from build123d import *

# Parameters (mm, degrees)
SKETCH1_W           = 32
SKETCH1_H           = 32
BOSS_EXTRUDE1_DEPTH = 5
BOSS_EXTRUDE2_DEPTH = 30
SKETCH3_R           = 5
SKETCH3_R_2         = 2
CUT_EXTRUDE1_DEPTH  = 10
SKETCH4_R           = 2
CUT_EXTRUDE2_DEPTH  = 58.210138962


with BuildPart() as part:
    # Sketch1 → Boss-Extrude1 (new body)
    with BuildSketch(Plane(origin=(0, 0, 0), x_dir=(1, 0, 0), z_dir=(0, 1, 0))):
        with Locations((0, -16)):
            Rectangle(SKETCH1_W, SKETCH1_H)
    extrude(amount=BOSS_EXTRUDE1_DEPTH)

    # Sketch2 → Boss-Extrude2 (add)
    with BuildSketch(Plane(origin=(0, 5, 0), x_dir=(1, 0, 0), z_dir=(0, 1, 0))):
        with BuildLine():
            Line((-16, -7), (-11.720842953, -7))
            ThreePointArc((-11.720842953, -7), (-11.587559316, -8.18927833), (-11, -9.231833616))
            Line((-11, -9.231833616), (-11, -22.772628888))
            ThreePointArc((-11, -22.772628888), (-11.586870055, -23.813052847), (-11.721238688, -25))
            Line((-11.721238688, -25), (-16, -25))
            Line((-16, -25), (-16, -7))
        make_face()
        with BuildLine():
            Line((16, -25), (11.725701193, -25))
            ThreePointArc((11.725701193, -25), (11.590282481, -23.809816196), (11, -22.767490763))
            Line((11, -22.767490763), (11, -9.236971742))
            ThreePointArc((11, -9.236971742), (11.590974158, -8.192515764), (11.725305458, -7))
            Line((11.725305458, -7), (16, -7))
            Line((16, -7), (16, -25))
        make_face()
    extrude(amount=BOSS_EXTRUDE2_DEPTH)

    # Sketch3 → Cut-Extrude1 (cut)
    with BuildSketch(Plane.XZ):
        with Locations(Location((0, 16, 0), (0, 0, 270))):
            Circle(SKETCH3_R)
        with Locations(Location((-8.732768748, 7.267231252, 0), (0, 0, 270))):
            Circle(SKETCH3_R_2)
        with Locations(Location((-8.732768748, 24.732768748, 0), (0, 0, 270))):
            Circle(SKETCH3_R_2)
        with Locations(Location((8.732768748, 24.732768748, 0), (0, 0, 270))):
            Circle(SKETCH3_R_2)
        with Locations(Location((8.732768748, 7.267231252, 0), (0, 0, 270))):
            Circle(SKETCH3_R_2)
    extrude(amount=-CUT_EXTRUDE1_DEPTH, mode=Mode.SUBTRACT)

    # Sketch4 → Cut-Extrude2 (cut, through all)
    with BuildSketch(Plane.ZY.offset(16)):
        with Locations((16, 23.5)):
            Circle(SKETCH4_R)
    extrude(amount=-CUT_EXTRUDE2_DEPTH, mode=Mode.SUBTRACT)


solid = part.part
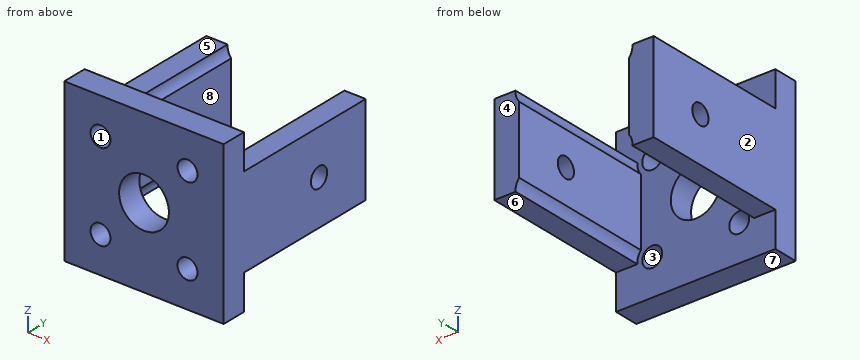
The listing builds one solid part. Answer for the finished solid, in the listing's coordinates (mm). Face numbers are marked on the shaded views. A direction names the side the tool comes from. Round coordinates to 2 decimals unless told otherwise and drop trailing zeros. Loops run counter-clockwise (first coordinate to the right, second up) from the corner with the lowest first, then second, coordinate; pieces in that order, holes last. Notation, with made-up numbers: M 73,57 L 113,57 A22 cw 113,72 Z; hole C -16.75,18.25 d8. An arc over 180 degrees is marked long. Return JSON: item names as keys, results as strings.
Q1. Find section A-A, the plane y = 23.5. Determine the outline of the cut face in (x, z).
Results list:
{"outline": "M -16,7 L -11.72,7 A3 cw -11,9.23 L -11,14 L -16,14 Z; M -16,18 L -11,18 L -11,22.77 A3 cw -11.72,25 L -16,25 Z; M 11,9.24 A3 cw 11.73,7 L 16,7 L 16,14 L 11,14 Z; M 11,18 L 16,18 L 16,25 L 11.73,25 A3 cw 11,22.77 Z"}
Q2. Each of these flat-tipped pins is pushed along its axis until it touches: pin 1 Ø8 at (x, z) = (0, 16) entering from +Y; pin 2 Ø1.3 at (x, y) = (13, 25.5) entering from +Z; pin 3 Ø4.5 at (x, z) = (-8.73, 24.73) entering from +Y; pin 4 Ø12 at (x, y) = (5.5, 21.5) entering from -Z. Where does it stop, or does it pass through?
Results list:
{"pin 1": "passes through", "pin 2": "stops at z = 25", "pin 3": "stops at y = 5", "pin 4": "stops at z = 8.44"}
Q3. Find section B-B, the plane x = 0. Determine the outline of the cut face in (y, z).
Results list:
{"outline": "M 0,0 L 5,0 L 5,11 L 0,11 Z; M 0,21 L 5,21 L 5,32 L 0,32 Z"}
Q4. The mould has two halves that part along X. Classify the marked faces 1, 2, 3 and 4: released by +X, released by -X, zero draft, split by the parting line, or undercut.
Results list:
{"face 1": "undercut", "face 2": "released by -X", "face 3": "undercut", "face 4": "zero draft"}
Q5. Find the intervals of material crossed by line 1 along X through (y, z) = (18, 12); line 2 along Z through (x, y) = (2, 2.5); line 3 along Y through (x, z) = (12.6, 16), in increasing order. Write a range as from..to.
Results list:
{"line 1": "x = -16..-11, 11..16", "line 2": "z = 0..11.42, 20.58..32", "line 3": "y = 0..21.5, 25.5..35"}
Q6. Find section D-D, the plane y = 12. Determine the outline of the cut face in (x, z), plus the area to 3 significant figures.
Results list:
{"outline": "M -16,7 L -11.72,7 A3 cw -11,9.23 L -11,22.77 A3 cw -11.72,25 L -16,25 Z; M 11,9.24 A3 cw 11.73,7 L 16,7 L 16,25 L 11.73,25 A3 cw 11,22.77 Z", "area": "175 mm2"}
Q7. Find section C-C, the plane z = 16. Determine the outline of the cut face in (x, y), plus the area to 3 significant figures.
Results list:
{"outline": "M -16,0 L -5,0 L -5,5 L -11,5 L -11,21.5 L -16,21.5 Z; M -16,25.5 L -11,25.5 L -11,35 L -16,35 Z; M 5,0 L 16,0 L 16,21.5 L 11,21.5 L 11,5 L 5,5 Z; M 11,25.5 L 16,25.5 L 16,35 L 11,35 Z", "area": "370 mm2"}
Q8. Which of the six approach directions +Z, -Z, +X, -X, +Y, -Y give full straight-line access (tool end or side, diameter ignored) to the marked faces 5, 6, 7 and 8?
Results list:
{"face 5": "+Z, +X, -X, +Y", "face 6": "-Z, +X, -X, +Y", "face 7": "-Z, +X, -X, +Y, -Y", "face 8": "+Z, -Z, +Y"}
